```python
from build123d import *

# Parameters (mm, degrees)
BOSS_EXTRUDE1_DEPTH      = 110
SHELL1_T                 = -2
BOSS_EXTRUDE2_REACH      = 172.36
BOSS_EXTRUDE2_END_RADIUS = 202


with BuildPart() as part:
    # Sketch1 → Boss-Extrude1 (new body)
    with BuildSketch(Plane.XY):
        with BuildLine():
            Line((-105, 181.865334795), (-100, 173.205080757))
            ThreePointArc((-100, 173.205080757), (0, 200), (100, 173.205080757))
            Line((100, 173.205080757), (105, 181.865334795))
            ThreePointArc((105, 181.865334795), (0, 210), (-105, 181.865334795))
        make_face()
    extrude(amount=-BOSS_EXTRUDE1_DEPTH)

    # Shell1
    shell1_openings = [part.faces().sort_by_distance(p)[0] for p in [
        (0, 210, -55),
    ]]
    offset(amount=SHELL1_T, openings=shell1_openings, kind=Kind.INTERSECTION)

    # Boss-Extrude2: up to this cylinder (the profile starts outside it)
    boss_extrude2_end = Plane(origin=(0, 0, -55), z_dir=(0, 0, 1)) * Cylinder(BOSS_EXTRUDE2_END_RADIUS, 749.72, mode=Mode.PRIVATE)
    # Sketch2 → Boss-Extrude2 (add, up to the surface)
    with BuildSketch(Plane(origin=(0, 250, 0), x_dir=(1, 0, 0), z_dir=(0, 1, 0)), mode=Mode.PRIVATE) as boss_extrude2_sk1:
        with BuildLine():
            ThreePointArc((-65.897237959, 35.122057745), (-83.691016821, 55), (-65.897237959, 74.877942255))
            ThreePointArc((-65.897237959, 74.877942255), (0, 75.948538311), (64.929649868, 64.646648447))
            ThreePointArc((64.929649868, 64.646648447), (72.294849357, 55), (64.929649868, 45.353351553))
            ThreePointArc((64.929649868, 45.353351553), (0, 34.051461689), (-65.897237959, 35.122057745))
        make_face()
    boss_extrude2_tool1 = extrude(boss_extrude2_sk1.sketch, amount=-BOSS_EXTRUDE2_REACH, mode=Mode.PRIVATE) - boss_extrude2_end
    add(boss_extrude2_tool1.solids().sort_by_distance((-11.41561, 250, -55))[0])


solid = part.part
```
Check sheet for the modelled part. Datum: model origin and axes. Units: mm. A direction names the side the tool comes from. Round coordinates to 2 decimals unless told otherwise and drop trailing zeros. Loops run counter-clockwise (first coordinate to the right, second up) from the corner with the lowest first, then second, coordinate; pieces in that order, holes last. Notation, with made-up numbers: (45.25, 42.25) - (104.25, 42.25) arc R16 ccw to (104.25, 49.25) - close; hole circle Ø5 at (85, 69.5). An arc over 180 degrees is marked (long way). Write item = value, one per line. Start each with the question number.
Q1. Section check D-D (y = 225.5). Record the boundary of the cut face in (x, z), plus the area to 3 significant figures.
Q2. Depth check by flat-ended pin: P1, Ø4, axis at x = 40.5, z = -94, coming from the +Y side; P2, Ø1, axis at x = -16, y = 233, coming from the -Z side; P3, Ø8, axis at x = 28, y = 216.5, coming from the -Z side. Enter the tip coordinate at first touch or a pass-through.
Q3. Access from +Z, -Z, +X, -X, +Y, -Y to the whole of each face (thin tool, end or side, straight path). Record for faces 1 (the face through (-83.687, 217.387, -54.591)), 2 (the face through (-0.92, 227.45, -76.02)), 3 (the face through (72.293, 219.74, -55.183)).
Q4. Thickness scan on L1, parallel to Z at x = 41, y = 202; L2, parallel to X at y = 180, z = -46; L3, parallel to Z at x = 65, y = 230. Record the ranges inside material, lowest first.
Q5. Section check C-C (x = 78). Record the boundary of the cut face in (y, z), plus the area to 3 significant figures.
Q6. Section check B-B (z = -17.5). Record the boundary of the cut face in (x, y).
Derived:
q1.outline = (-65.9, -74.88) arc R350 ccw to (64.93, -64.65) arc R10 ccw to (64.93, -45.35) arc R350 ccw to (-65.9, -35.12) arc R20 ccw to start
q1.area = 5,600 mm^2
q2.P1 = 198.3
q2.P2 = -76.85
q2.P3 = -73.24
q3.face_1 = -X, +Y
q3.face_2 = +Y
q3.face_3 = +X, +Y
q4.L1 = -110 to -108, -70.29 to -39.71, -2 to 0
q4.L2 = -103.92 to -101.61, -91.67 to -87.18, 87.18 to 91.67, 101.61 to 103.92
q4.L3 = -64.63 to -45.37
q5.outline = (184.16, -110) - (194.98, -110) - (194.98, -108) - (186.33, -108) - (186.33, -2) - (194.98, -2) - (194.98, 0) - (184.16, 0) - close
q5.area = 273 mm^2
q6.outline = (-105, 181.87) - (-100, 173.21) arc R200 cw to (100, 173.21) - (105, 181.87) arc R210 ccw to (103.26, 182.86) - (99.26, 175.93) arc R202 ccw to (-99.26, 175.93) - (-103.26, 182.86) arc R210 ccw to start
